Verification items for the finished model (mm, model axes). Give positions to 0.01 mm unless a question says otherwise; leave off trailing zeros. Write each loop counter-clockwise with the first axis right and the second up, starting at its lowest first coordinate (ties: lowest second). Pieces come first, ordered by that corner, then holes. Notation, with made-up numbers: (89.25, 69.5) -> (117.25, 69.5) arc R24 ccw to (117.25, 96.5) -> close; hole circle Ø8 at (42, 78.5). An arc over 180 degrees is marked (long way). Answer as CSV lines item,"result".
```python
from build123d import *

# Parameters (mm, degrees)
F0_R     = 1
F0_W     = 8
F0_H     = 20
F1_DEPTH = 3


with BuildPart() as f1:
    # F0 (on Front) → F1 (new body)
    with BuildSketch(Plane.XZ):
        with BuildLine():
            Line((23, 1e-06), (1, 0))
            ThreePointArc((1, 0), (0.292893, -0.292893), (0, -1))
            Line((0, -1), (0, -23.999999))
            ThreePointArc((0, -23.999999), (0.292893, -24.707106), (1, -24.999999))
            Line((1, -24.999999), (6, -24.999999))
            ThreePointArc((6, -24.999999), (6.707107, -25.292892), (7, -25.999999))
            Line((7, -25.999999), (7, -33.999999))
            ThreePointArc((7, -33.999999), (8, -34.999999), (7, -35.999999))
            Line((7, -35.999999), (7, -43.999999))
            ThreePointArc((7, -43.999999), (7.292893, -44.707106), (8, -44.999999))
            Line((8, -44.999999), (16, -44.999999))
            ThreePointArc((16, -44.999999), (16.707107, -44.707106), (17, -43.999999))
            Line((17, -43.999999), (17, -35.999999))
            ThreePointArc((17, -35.999999), (16, -34.999999), (17, -33.999999))
            Line((17, -33.999999), (17, -25.999999))
            ThreePointArc((17, -25.999999), (17.292893, -25.292892), (18, -24.999999))
            Line((18, -24.999999), (23, -24.999999))
            ThreePointArc((23, -24.999999), (23.707107, -24.707106), (24, -23.999999))
            Line((24, -23.999999), (24, -0.999999))
            ThreePointArc((24, -0.999999), (23.707107, -0.292892), (23, 1e-06))
        make_face()
        with Locations((1.5, -22.999999)):
            Circle(F0_R, mode=Mode.SUBTRACT)
        with Locations((22.5, -22.999999)):
            Circle(F0_R, mode=Mode.SUBTRACT)
        with Locations((1.5, -10.599999)):
            Circle(F0_R, mode=Mode.SUBTRACT)
        with Locations((12, -13)):
            Rectangle(F0_W, F0_H, mode=Mode.SUBTRACT)
        with Locations((22.5, -10.599999)):
            Circle(F0_R, mode=Mode.SUBTRACT)
    extrude(amount=F1_DEPTH)


solid = f1.part
```
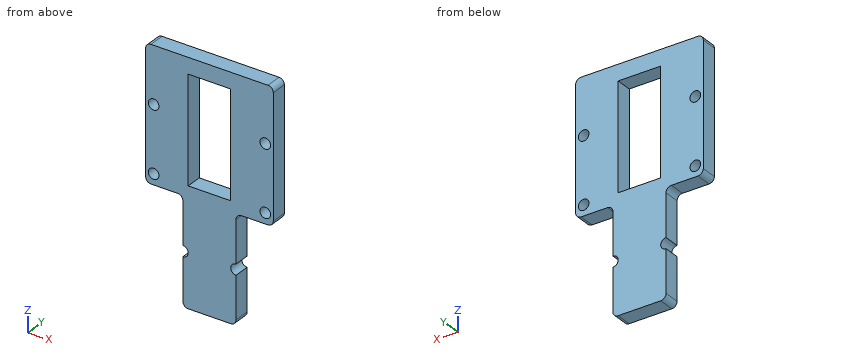
1) Section check C-C (y = -0.7). Record the boundary of the cut face in (x, z).
Reported:
outline,"(0, -24) arc R1 ccw to (1, -25) -> (6, -25) arc R1 cw to (7, -26) -> (7, -34) arc R1 cw to (7, -36) -> (7, -44) arc R1 ccw to (8, -45) -> (16, -45) arc R1 ccw to (17, -44) -> (17, -36) arc R1 cw to (17, -34) -> (17, -26) arc R1 cw to (18, -25) -> (23, -25) arc R1 ccw to (24, -24) -> (24, -1) arc R1 ccw to (23, 0) -> (1, 0) arc R1 ccw to (0, -1) -> close; hole circle Ø2 at (1.5, -23); hole circle Ø2 at (1.5, -10.6); hole (8, -23) -> (16, -23) -> (16, -3) -> (8, -3) -> close; hole circle Ø2 at (22.5, -23); hole circle Ø2 at (22.5, -10.6)"
2) Section check D-D (x = 11). Record the boundary of the cut face in (y, z).
Reported:
outline,"(-3, -45) -> (0, -45) -> (0, -23) -> (-3, -23) -> close; (-3, -3) -> (0, -3) -> (0, 0) -> (-3, 0) -> close"
3) Depth check by flat-ended pin: pin 1 (1.5 mm diameter, centred on y = -1.5, z = -28.5, fed in from +X); pin 2 (1.5 mm diameter, centred on x = 20.5, y = -1, fed in from -Z); pin 3 (3 mm diameter, centred on x = 1.5, z = -10.6, fed in from +Y); pin 4 (0.9 mm diameter, centred on y = -1.5, z = -38.5, fed in from -X). Enter the tip coordinate at first touch or a pass-through.
Reported:
pin 1,"x = 17"
pin 2,"z = -25"
pin 3,"y = 0"
pin 4,"x = 7"
4) Scan lines: line 1 along Z through (x, y) = (1.5, -1.45); line 2 along X through (y, z) = (-2.6, -5.5); line 3 along Z through (x, y) = (12.5, -0.65). Record each from-to range of solid material in increasing order.
Reported:
line 1,"-25 to -24, -22 to -11.6, -9.6 to 0"
line 2,"0 to 8, 16 to 24"
line 3,"-45 to -23, -3 to 0"
5) Section check B-B (z = -13). Record the boundary of the cut face in (x, y).
Reported:
outline,"(0, -3) -> (8, -3) -> (8, 0) -> (0, 0) -> close; (16, -3) -> (24, -3) -> (24, 0) -> (16, 0) -> close"
6) Section check A-A (x = 22.5). Record the boundary of the cut face in (y, z).
Reported:
outline,"(-3, -25) -> (0, -25) -> (0, -24) -> (-3, -24) -> close; (-3, -22) -> (0, -22) -> (0, -11.6) -> (-3, -11.6) -> close; (-3, -9.6) -> (0, -9.6) -> (0, 0) -> (-3, 0) -> close"
